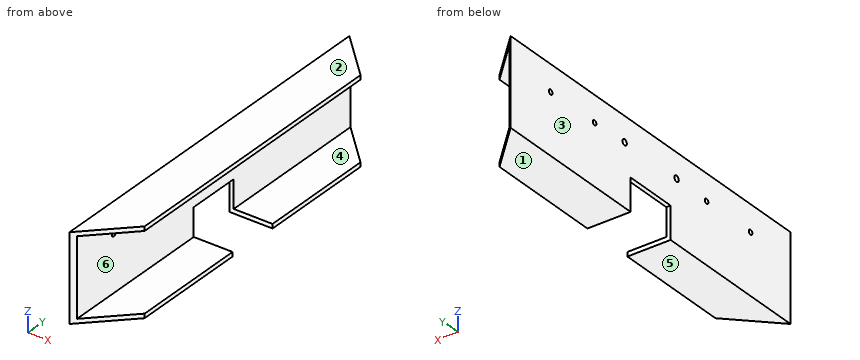
Solid Edge part; units mm, degrees
sketch "Sketch1" plane through (0, 0, 0) normal (0, -1, 0) x (1, 0, 0)
  line L0 (20, 36) -> (-16, 36)
  line L1 (-16, 36) -> (-16, -36)
  line L2 (-16, -36) -> (20, -36)
  line L3 (20, -36) -> (20, -40)
  line L4 (20, -40) -> (-20, -40)
  line L5 (-20, -40) -> (-20, 40)
  line L6 (-20, 40) -> (20, 40)
  line L7 (20, 40) -> (20, 36)
  dimension "D1" = 20
  dimension "D2" = 20
  dimension "D3" = 20
extrude "Protrusion1" add sketch "Sketch1" against normal blind 350
sketch "Sketch2" plane through (0, 175, 40) normal (0, 0, 1) x (0, 1, 0)
  line L0 (-175, 20) -> (-135, -20)
extrude "Cutout1" cut sketch "Sketch2" against normal through all material side at (0.0354, 19.9646, 40)
sketch "Sketch3" plane through (0, 175, 40) normal (0, 0, 1) x (0, 1, 0)
  line L0 (175, 20) -> (135, -20)
extrude "Cutout2" cut sketch "Sketch3" against normal through all material side at (0.0354, 330.0354, 40)
hole "Bohrung_1" at (-16, 142.5, 17) direction (-1, 0, 0) diameter 5.5 end up to next
hole "Hole1" at (-16, 207.5, 17) direction (-1, 0, 0) diameter 5.5 end up to next
hole "Bohrung_3" at (-16, 50, 15.6) direction (-1, 0, 0) diameter 4.5 end up to next
hole "Hole2" at (-16, 105, 15.6) direction (-1, 0, 0) diameter 4.5 end up to next
hole "Hole3" at (-16, 245, 15.6) direction (-1, 0, 0) diameter 4.5 end up to next
hole "Hole4" at (-16, 300, 15.6) direction (-1, 0, 0) diameter 4.5 end up to next
sketch "Sketch4" plane through (20, 175, -38) normal (1, 0, 0) x (0, 1, 0)
  line L0 (-25, -2) -> (25, -2)
  line L1 (25, -2) -> (25, 28)
  line L2 (25, 28) -> (-25, 28)
  line L3 (-25, 28) -> (-25, -2)
  dimension "D1" = 25
  dimension "D2" = 25
extrude "Cutout3" cut sketch "Sketch4" against normal through all
Design review of the part built by this model. Coordinates are the model's own, in mm. Face numbers are marked on the shaded views. A direction names the side the tool comes from. Round coordinates to 2 decimals unless told otherwise and drop trailing zeros. Write each loop counter-clockwise with the first axis right and the second up, starting at its lowest first coordinate (ties: lowest second). Pieces come first, ordered by that corner, then holes.
Item 1: Draft analysis for pull direction Z (two halves, no side actions). For the marked faces 1, 2, 3 and 4, state which applies: released by +Z, released by -Z, zero draft, split by the parting line, or undercut.
Item 2: Consider section C-C on y = 125. Give the boundary of the cut face in (x, z).
Item 3: Consider section B-B on z = -30.5. Give the boundary of the cut face in (x, y).
Item 4: Wall thickness on L1, parallel to Z at x = 6, y = 130; L2, parallel to Z at x = -18, y = 207; L3, parallel to X at y = 20, z = 12.5: over which ranges is each line inside the solid? List them lowest first.
Item 5: For pin 1 Ø21.5 at (y, z) = (214.5, -0.5) entering from +X; pin 2 Ø4 at (y, z) = (50, 15.6) entering from -X; pin 3 Ø4.5 at (x, y) = (-17.5, 180) entering from -Z, all flat-tipped, find the tip position at first contact; note any pin that passes through.
Item 6: Consider section A-A on x = -1. Give the boundary of the cut face in (y, z), and give its area (3 significant figures).
Item 7: Consider section D-D on y = 185. Give the boundary of the cut face in (x, z).
Item 8: For the marked faces 5 and 6, list the 3-axis set-ups (+Z, -Z, +X, -X, +Y, -Y) from which the entire face can be reached by the end or side of a thin tool; tool diameter is ignored.
Check values:
1. face 1: released by -Z
1. face 2: released by +Z
1. face 3: zero draft
1. face 4: undercut
2. outline: (-20, -40) - (20, -40) - (20, -36) - (-16, -36) - (-16, 36) - (20, 36) - (20, 40) - (-20, 40) - close
3. outline: (-20, 0) - (-16, 4) - (-16, 150) - (-20, 150) - close; (-20, 200) - (-16, 200) - (-16, 346) - (-20, 350) - close
4. L1: z = -40 to -36, 36 to 40
4. L2: z = -40 to 14.3, 19.7 to 40
4. L3: x = -20 to -16
5. pin 1: stops at x = -16
5. pin 2: passes through
5. pin 3: stops at z = -10
6. outline: (19, -40) - (150, -40) - (150, -36) - (19, -36) - close; (19, 36) - (331, 36) - (331, 40) - (19, 40) - close; (200, -40) - (331, -40) - (331, -36) - (200, -36) - close
6. area: 2,300 mm2
7. outline: (-20, -10) - (-16, -10) - (-16, 36) - (20, 36) - (20, 40) - (-20, 40) - close
8. face 5: -Z, +X, -X, +Y, -Y
8. face 6: +X, +Y, -Y
